```python
from build123d import *

# Parameters (mm, degrees)
F1_DEPTH = 67
F3_DEPTH = 60
F5_R     = 35
F6_DEPTH = 7


with BuildPart() as f1:
    # F0 (on Front) → F1 (new body)
    with BuildSketch(Plane.XZ):
        with BuildLine():
            Line((-115, 70), (-124.666667, 70))
            ThreePointArc((-124.666667, 70), (-190, 0), (-124.666667, -70))
            Line((-124.666667, -70), (-115, -70))
            Line((-115, -70), (115, -70))
            Line((115, -70), (124.666667, -70))
            ThreePointArc((124.666667, -70), (190, 0), (124.666667, 70))
            Line((124.666667, 70), (115, 70))
            Line((115, 70), (-115, 70))
        make_face()
    extrude(amount=-F1_DEPTH)

    # F2 (on face) → F3 (cut)
    with BuildSketch(Plane.XZ):
        with BuildLine():
            ThreePointArc((-114.5, 69.5), (-119.798333, 69.701667), (-125.096667, 69.5))
            Line((-125.096667, 69.5), (-114.5, 69.5))
        make_face()
        with BuildLine():
            Line((-114.5, 69.5), (-125.096667, 69.5))
            ThreePointArc((-125.096667, 69.5), (-189.5, 0), (-125.096667, -69.5))
            Line((-125.096667, -69.5), (-114.5, -69.5))
            Line((-114.5, -69.5), (114.5, -69.5))
            Line((114.5, -69.5), (125.096667, -69.5))
            ThreePointArc((125.096667, -69.5), (189.5, 0), (125.096667, 69.5))
            Line((125.096667, 69.5), (114.5, 69.5))
            Line((114.5, 69.5), (-114.5, 69.5))
        make_face()
        with BuildLine():
            Line((-114.5, -69.5), (-125.096667, -69.5))
            ThreePointArc((-125.096667, -69.5), (-119.798333, -69.701667), (-114.5, -69.5))
        make_face()
        with BuildLine():
            ThreePointArc((125.096667, 69.5), (119.798333, 69.701667), (114.5, 69.5))
            Line((114.5, 69.5), (125.096667, 69.5))
        make_face()
        with BuildLine():
            Line((125.096667, -69.5), (114.5, -69.5))
            ThreePointArc((114.5, -69.5), (119.798333, -69.701667), (125.096667, -69.5))
        make_face()
    extrude(amount=-F3_DEPTH, mode=Mode.SUBTRACT)

    # F4: F1 across face


with BuildPart() as f1_1:
    add(f1.part)
    add(f1.part.mirror(Plane.XZ))

    # F5 (on face) → F6 (cut, through all)
    with BuildSketch(Plane.XZ.offset(67)):
        with Locations((-114.5, 0)):
            Circle(F5_R)
        with Locations((114.5, 0)):
            Circle(F5_R)
    extrude(amount=-F6_DEPTH, mode=Mode.SUBTRACT)


solid = f1_1.part
```
For this review, take the finished solid that the model builds, in its own axes (mm). A direction names the side the tool comes from. Coordinates: 2 decimals unless noted, no trailing zeros. Loops run counter-clockwise (first coordinate to the right, second up) from the corner with the lowest first, then second, coordinate; pieces in that order, holes last.
1. For line 1 (Y direction, x = -72.5, z = 49); line 2 (Z direction, x = -53.5, y = -33); line 3 (Z direction, x = 114, y = -64), list the stretches that pass through material, from the lowest coordinate up.
2. Mouldability with a two-part tool opening along Z and no side actions: class faces 1 (the flat face through (-3, 60, 1)), 2 (the flat face through (-3, -67, 1)), 3 (the flat face through (-2, 1, -70)), 4 (the cylindrical face through (119.7, 0.8, -69.7)) as +Z half, -Z half, draft (parallel to the pull), parting line (faces both ways), or undercut.
3. For faces 5 (the cylindrical face through (-189.984, 0.938, 1.475)), 6 (the flat face through (-2, 1, -69.5)), 7 (the cylindrical face through (-82.17, -63.55, -13.41)), list the 3-axis set-ups (+Z, -Z, +X, -X, +Y, -Y) from which the entire face can be reached by the end or side of a thin tool; tool diameter is ignored.
4. Add section D-D, the plane z = 49. Give the boundary of the cut face in (x, y), then the cut area to 3 significant figures.
5. Add section A-A, the plane x = -59. Give the boundary of the cut face in (y, z), then the cut area to 3 significant figures.
6. Insertion check: P1, Ø12, axis at y = 29.5, z = -49, coming from the -X side; P2, Ø3, axis at y = -14, z = -23, coming from the -X side; P3, Ø2, axis at x = -136.5, y = -49, coming from the -Z side. Each pin has a flat end and moves straight along its axis. Give the tip position at first contact, or say it passes through.
7. Add section B-B, the plane z = 0. Give the boundary of the cut face in (x, y), then the cut area to 3 significant figures.
8. Add section C-C, the plane y = -3.5. Give the boundary of the cut face in (x, z).
Result:
1. line 1: y = -67 to -60, 60 to 67
1. line 2: z = -70 to -69.5, 69.5 to 70
1. line 3: z = -70 to -35, 35 to 70
2. face 1: undercut
2. face 2: draft
2. face 3: -Z half
2. face 4: undercut
3. face 5: -X, +Y, -Y
3. face 6: none
3. face 7: -Y
4. outline: (-170.06, -67) - (170.06, -67) - (170.06, 67) - (-170.06, 67) - close; hole (-169.37, -60) - (169.37, -60) - (169.37, 60) - (-169.37, 60) - close
4. area: 4,930 mm2
5. outline: (-67, -70) - (67, -70) - (67, 70) - (-67, 70) - close; hole (-60, -69.5) - (60, -69.5) - (60, 69.5) - (-60, 69.5) - close
5. area: 2,080 mm2
6. P1: stops at x = -175.28
6. P2: stops at x = -186.62
6. P3: stops at z = -68.4
7. outline: (-190, -67) - (-149.5, -67) - (-149.5, -60) - (-189.5, -60) - (-189.5, 60) - (189.5, 60) - (189.5, -60) - (149.5, -60) - (149.5, -67) - (190, -67) - (190, 67) - (-190, 67) - close; (-79.5, -67) - (79.5, -67) - (79.5, -60) - (-79.5, -60) - close
7. area: 4,460 mm2
8. outline: (-124.67, -70) - (124.67, -70) arc R70.17 ccw to (124.67, 70) - (-124.67, 70) arc R70.17 ccw to start; hole (-125.1, -69.5) arc R69.7 ccw to (-114.5, -69.5) - (114.5, -69.5) arc R69.7 ccw to (125.1, -69.5) arc R69.7 ccw to (125.1, 69.5) arc R69.7 ccw to (114.5, 69.5) - (-114.5, 69.5) arc R69.7 ccw to (-125.1, 69.5) arc R69.7 ccw to start
